Can you work these out from the model? Positions are in its coordinate system, mm. Face numbers are marked on the shaded views. A direction names the side the tool comes from. Coordinates: 2 decimals unless noted, no trailing zeros. Loops run counter-clockwise (first coordinate to the right, second up) from the corner with the lowest first, then second, coordinate; pieces in that order, holes last.
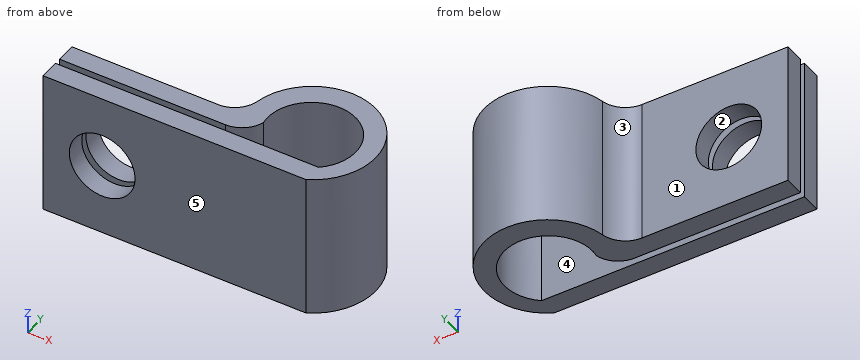
```python
from build123d import *

# Parameters (mm, degrees)
SKETCH1_W           = 14.546192004
SKETCH1_H           = 1.5
SKETCH1_W_2         = 20
BOSS_EXTRUDE1_DEPTH = 11
SKETCH2_R           = 2.5
CUT_EXTRUDE1_DEPTH  = 25.55732176
FILLET1_R           = 2


with BuildPart() as part:
    # Sketch1 → Boss-Extrude1 (new body)
    with BuildSketch(Plane.XY):
        with Locations((-12.726903998, 2.75)):
            Rectangle(SKETCH1_W, SKETCH1_H)
        with BuildLine():
            Line((0, 1.5), (0, 0))
            ThreePointArc((0, 0), (-0.056155977, 8.546349982), (-6.953807996, 3.5))
            Line((-6.953807996, 3.5), (-5.453807996, 3.5))
            ThreePointArc((-5.453807996, 3.5), (-0.998787688, 7.212407275), (0, 1.5))
        make_face()
        with Locations((-10, 0.75)):
            Rectangle(SKETCH1_W_2, SKETCH1_H)
    extrude(amount=BOSS_EXTRUDE1_DEPTH)

    # Sketch2 → Cut-Extrude1 (cut, through all)
    with BuildSketch(Plane(origin=(0, 0, 0), x_dir=(-1, 0, 0), z_dir=(0, -1, 0))):
        with Locations(Location((15.5, -5.5, 0), (0, 0, 270))):
            Circle(SKETCH2_R)
    extrude(amount=-CUT_EXTRUDE1_DEPTH, mode=Mode.SUBTRACT)

    # Fillet1
    # the kernel refuses this fillet: 2 mm, written as the material it adds along each edge
    with BuildSketch(Plane(origin=(-6.953807996, 3.5, 0), x_dir=(-1, 0, 0), z_dir=(0, 0, 1))) as fillet1_piece_1:
        with BuildLine():
            CenterArc((1.946122673, -2), FILLET1_R, 90, 79.482966368)
            ThreePointArc((-0.0202787, -1.634944336), (0.059988825, -0.818341988), (0, 0))
            Line((0, 0), (1.946122673, 0))
        make_face()
    extrude(amount=11)
    # the kernel refuses this fillet: 2 mm, written as the material it takes off along each edge
    with BuildSketch(Plane(origin=(-5.453807996, 2, -4.841229183), x_dir=(-1, 0, 0), z_dir=(0, 0, 1))) as fillet1_2_piece_1:
        with BuildLine():
            CenterArc((1.936491673, -2), FILLET1_R, 90, 75.522487814)
            Line((0, -1.5), (0, 0))
            Line((0, 0), (1.936491673, 0))
        make_face()
    extrude(amount=20.682458366, mode=Mode.SUBTRACT)


solid = part.part
```
Item 1: Suppose I cut it at A-A, the plane z = 5.5. Please give me the cut outline in (x, y), plus the area to 3 significant figures.
Results are:
outline: (-20, 0) - (-18, 0) - (-18, 1.5) - (-20, 1.5) - close; (-20, 2) - (-18, 2) - (-18, 3.5) - (-20, 3.5) - close; (-13, 0) - (0, 0) arc R4.8 ccw (long way) to (-6.93, 5.13) arc R2 cw to (-8.9, 3.5) - (-13, 3.5) - (-13, 2) - (-7.39, 2) arc R2 ccw to (-5.45, 3.5) arc R3.35 cw (long way) to (0, 1.5) - (-13, 1.5) - close
area: 63.3 mm2
Item 2: I'm going to push a flat-ended pin straight in: P1, Ø6.5, axis at x = -15.5, z = 5.5, coming from the +Y side. Where does the tip first touch, or does it pass through?
Results are:
P1: stops at y = 3.5
Item 3: On a 3-axis mill with a long thin cutter (end or side, diameter ignored), from which of +Z, -Z, +X, -X, +Y, -Y can I reach the whole of each face in a straight line? I mean the marked faces 4 and 5. Say none if no direction works.
Results are:
face 4: +Z, -Z, -X
face 5: +Z, -Z, +X, -X, -Y
Item 4: Suppose I cut it at D-D, the plane x = -15.5. Please give me the cut outline in (y, z).
Results are:
outline: (0, 0) - (1.5, 0) - (1.5, 3) - (0, 3) - close; (0, 8) - (1.5, 8) - (1.5, 11) - (0, 11) - close; (2, 0) - (3.5, 0) - (3.5, 3) - (2, 3) - close; (2, 8) - (3.5, 8) - (3.5, 11) - (2, 11) - close
Item 5: I need wall thicknesses on line 1 along Z through (x, y) = (-15.5, 1.15); line 2 along Y through (x, z) = (-18.5, 3.25); line 3 along X through (y, z) = (2.7, 5.5). Which ranges of each line are inside material? Lowest first, please.
Results are:
line 1: z = 0 to 3, 8 to 11
line 2: y = 0 to 1.5, 2 to 3.5
line 3: x = -20 to -18, -13 to -5.87, 0.91 to 2.33
Item 6: Suppose I cut it at B-B, the plane y = 6. Please give me the cut outline in (x, z), plus the area to 3 significant figures.
Results are:
outline: (-6.69, 0) - (-4.89, 0) - (-4.89, 11) - (-6.69, 11) - close; (0.58, 0) - (2.26, 0) - (2.26, 11) - (0.58, 11) - close
area: 38.2 mm2
Item 7: Suppose I cut it at C-C, the plane x = 0.25. Please give me the cut outline in (y, z).
Results are:
outline: (0.14, 0) - (1.73, 0) - (1.73, 11) - (0.14, 11) - close; (6.4, 0) - (8.38, 0) - (8.38, 11) - (6.4, 11) - close
Item 8: We'd pull the mould along X, two halves only. Please class the marked faces 1, 2 and 3: +X half, -X half, draft (parallel to the pull), parting line (faces both ways), or undercut.
Results are:
face 1: draft
face 2: undercut
face 3: -X half
